```python
from build123d import *

# Parameters (mm, degrees)
BOSS_EXTRUDE1_DEPTH = 80
SKETCH2_R           = 30
CUT_EXTRUDE1_DEPTH  = 795.858645519
SKETCH4_R           = 97
BOSS_EXTRUDE3_DEPTH = 80
FILLET1_R           = 81.12


with BuildPart() as part:
    # Sketch1 → Boss-Extrude1 (new body)
    with BuildSketch(Plane.XY):
        with BuildLine():
            Line((-37.300835355, 250), (362.699164645, 250))
            ThreePointArc((362.699164645, 250), (612.699164645, 0), (362.699164645, -250))
            Line((362.699164645, -250), (-37.300835355, -250))
            ThreePointArc((-37.300835355, -250), (-287.300835355, 0), (-37.300835355, 250))
        make_face()
    extrude(amount=BOSS_EXTRUDE1_DEPTH)

    # Sketch2 → Cut-Extrude1 (cut, through all)
    with BuildSketch(Plane(origin=(0, 250, 0), x_dir=(1, 0, 0), z_dir=(0, 1, 0))):
        with Locations(Location((302.549396618, -40.40928544, 0), (0, 0, 270))):
            Circle(SKETCH2_R)
    extrude(amount=-CUT_EXTRUDE1_DEPTH, mode=Mode.SUBTRACT)

    # Sketch4 → Boss-Extrude3 (add)
    with BuildSketch(Plane(origin=(0, 0, 0), x_dir=(-1, 0, 0), z_dir=(0, 0, -1))):
        with Locations(Location((125.244285171, 0, 0), (0, 0, 180))):
            Circle(SKETCH4_R)
    extrude(amount=BOSS_EXTRUDE3_DEPTH)

    # Fillet1
    # the kernel refuses this fillet: 81.12 mm, written as the material it takes off along each edge
    with BuildSketch(Plane(origin=(-125.244285171, 0, -80), x_dir=(1, 0, 0), z_dir=(0, 1, 0))) as fillet1_piece_1:
        with BuildLine():
            CenterArc((15.887732124, -81.12), FILLET1_R, 0.791091124, 89.208908876)
            Line((15.887732124, 0), (15.887732124, 1.6224))
            Line((15.887732124, 1.6224), (97, 1.6224))
            Line((97, 1.6224), (98.6224, 0))
            ThreePointArc((98.6224, 0), (98.6224, -40), (98.622245358, -79.9776))
            Line((98.622245358, -79.9776), (97, -80))
        make_face()
    revolve(axis=Axis((-125.244285171, 0, -80), (0, 0, -1)), mode=Mode.SUBTRACT)


solid = part.part
```
For this review, take the finished solid that the model builds, in its own axes (mm). Round coordinates to 2 decimals unless told otherwise and drop trailing zeros. Write each loop counter-clockwise with the first axis right and the second up, starting at its lowest first coordinate (ties: lowest second). Pieces come first, ordered by that corner, then holes. Notation, with made-up numbers: M -15,46.5 L 36,46.5 A25 ccw 36,81.5 Z; hole C 30.25,-2 d7. An arc over 180 degrees is marked long. One line per item, written item: value. Start each with the question number.
(1) Insertion check: pin 1 (1 mm diameter, centred on x = -187.5, y = -88.5, fed in from -Z); pin 2 (8 mm diameter, centred on y = -134, z = 13, fed in from -X); pin 3 (2 mm diameter, centred on x = -97, z = 44.5, fed in from +Y). Each pin has a flat end and moves straight along its axis. Give the tip position at first contact, or say it passes through.
(2) We need section B-B (x = 82). Give the boundary of the cut face in (y, z).
(3) Wall thickness on line 1 (Z direction, x = 13, y = -168); line 2 (X direction, y = 194, z = 65); line 3 (X direction, y = -121.5, z = 59.5): over which ranges is each line inside the solid? List them lowest first.
(4) We need section A-A (z = 22). Give the boundary of the cut face in (x, y).
(5) The part is to be moulded in two halves that separate along X. For faces 1 (the cylindrical face through (275.934, 3.5, 54.252)), 2 (the flat face through (165, -250, 39)), 3 (the cylindrical face through (612.64, 5.5, 39.44)), say which applies: released by +X, released by -X, zero draft, split by the parting line, or undercut.
Result:
1. pin 1: z = 0
1. pin 2: x = -250.84
1. pin 3: y = 243.01
2. outline: M -250,0 L 250,0 L 250,80 L -250,80 Z
3. line 1: 0 to 80
3. line 2: -194.98 to 285.37, 319.73 to 520.38
3. line 3: -255.79 to 279.41, 325.69 to 581.19
4. outline: M -37.3,-250 L 278.86,-250 L 278.86,250 L -37.3,250 A250 ccw Z; M 326.24,-250 L 362.7,-250 A250 ccw 362.7,250 L 326.24,250 Z
5. face 1: undercut
5. face 2: zero draft
5. face 3: released by +X
